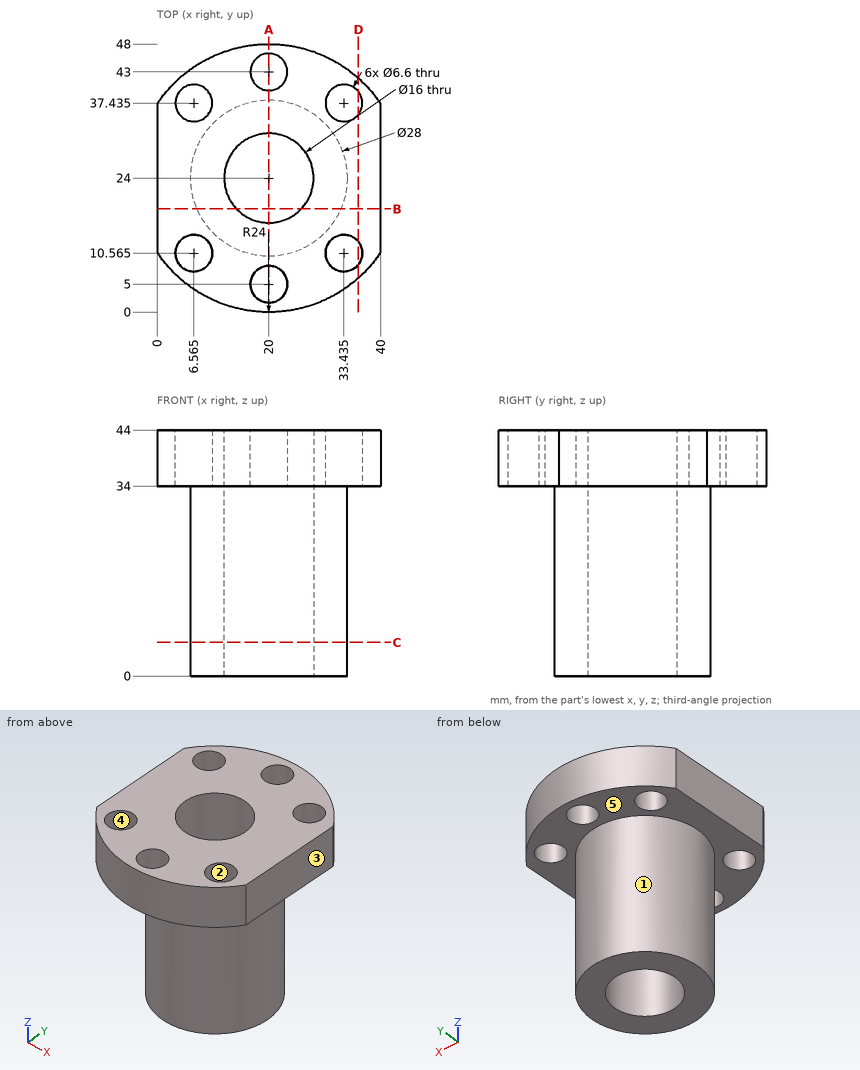
The drawing under review shows one solid part. Ordinate dimensions are in mm from its lowest x, y, z. A direction names the side the tool comes from. Coordinates: 2 decimals unless noted, no trailing zeros. Loops run counter-clockwise (first coordinate to the right, second up) from the corner with the lowest first, then second, coordinate; pieces in that order, holes last. Notation, with made-up numbers: (12, 19.5) - (69, 19.5) arc R30 cw to (69, 46.5) - close; hole circle Ø1 at (-20, 88). An arc over 180 degrees is marked (long way). Use CSV: the item, a comma, the result in double quotes. Start each with the question number.
1. Add section A-A on x = 20. Give the boundary of the cut face in (y, z).
2. For the marked faces 4 and 5, list the 3-axis set-ups (+Z, -Z, +X, -X, +Y, -Y) from which the entire face can be reached by the end or side of a thin tool; tool diameter is ignored.
3. Add section C-C on z = 6. Give the boundary of the cut face in (x, y), plus the area to 3 significant figures.
4. Add section B-B on y = 18.5. Give the boundary of the cut face in (x, z), plus the area to 3 significant figures.
5. To check wall thickness, follow probe 1 along Z at (x, y) = (10, 43); probe 2 along X at (y, z) = (10, 39); probe 3 along X at (y, z) = (23, 42). State the ranges of each line that lie inside material, in increasing order.
6. Mouldability with a two-part tool opening along X and no side actions: class the marked faces 1, 2 and 3 as released by +X, released by -X, zero draft, split by the parting line, or undercut.
7. Clearance check with flat-ended pins moving along their axes: pin 1 (5 mm diameter, centred on x = 18.5, z = 8.5, fed in from -Y); pin 2 (5 mm diameter, centred on x = 30.5, z = 13.5, fed in from -Y); pin 3 (18.5 mm diameter, centred on x = 20, y = 24, fed in from +Z); pin 4 (10 mm diameter, centred on x = 7, z = 20.5, fed in from +Y). State where each tip first meets the part, or that it passes through.
8. Add section D-D on x = 36. Give the boundary of the cut face in (y, z), plus the area to 3 significant figures.
Resolved:
1,outline,"(0, 34) - (1.7, 34) - (1.7, 44) - (0, 44) - close; (8.3, 34) - (10, 34) - (10, 0) - (16, 0) - (16, 44) - (8.3, 44) - close; (32, 0) - (38, 0) - (38, 34) - (39.7, 34) - (39.7, 44) - (32, 44) - close; (46.3, 34) - (48, 34) - (48, 44) - (46.3, 44) - close"
2,face 4,"+Z, -Z"
2,face 5,"-Z"
3,outline,"circle Ø28 at (20, 24); hole circle Ø16 at (20, 24)"
3,area,"415 mm2"
4,outline,"(0, 34) - (7.13, 34) - (7.13, 0) - (14.19, 0) - (14.19, 44) - (0, 44) - close; (25.81, 0) - (32.87, 0) - (32.87, 34) - (40, 34) - (40, 44) - (25.81, 44) - close"
4,area,"764 mm2"
5,probe 1,"34 to 44"
5,probe 2,"0.51 to 3.31, 9.82 to 30.18, 36.69 to 39.49"
5,probe 3,"0 to 12.06, 27.94 to 40"
6,face 1,"split by the parting line"
6,face 2,"undercut"
6,face 3,"released by +X"
7,pin 1,"y = 10"
7,pin 2,"y = 12.51"
7,pin 3,"z = 44"
7,pin 4,"y = 35.49"
8,outline,"(6.11, 34) - (8.49, 34) - (8.49, 44) - (6.11, 44) - close; (12.64, 34) - (35.36, 34) - (35.36, 44) - (12.64, 44) - close; (39.51, 34) - (41.89, 34) - (41.89, 44) - (39.51, 44) - close"
8,area,"275 mm2"
